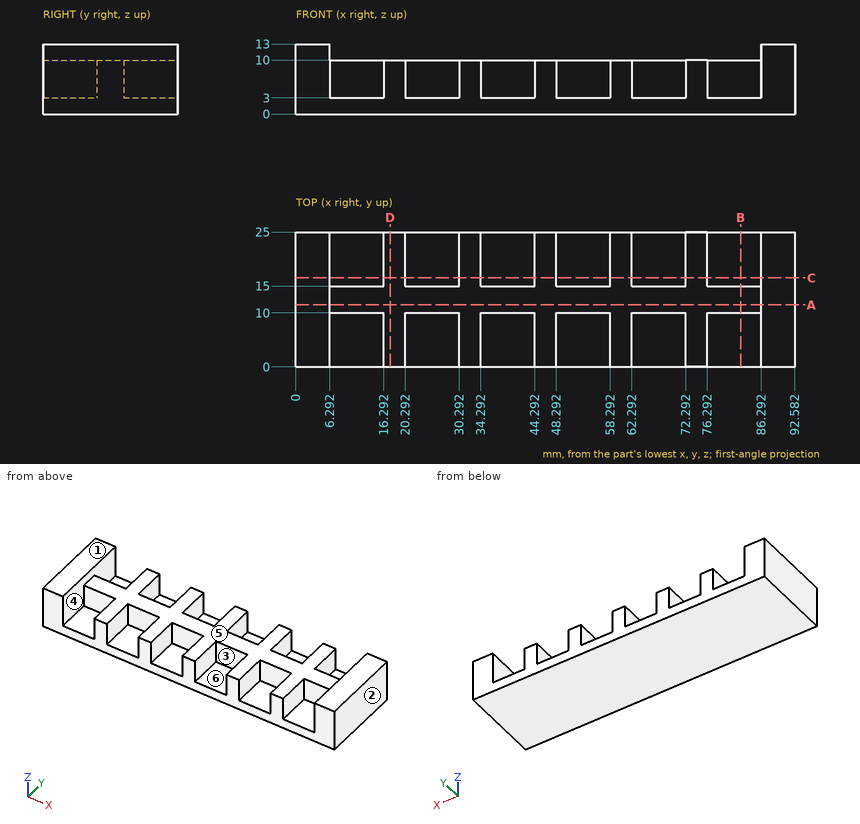
Part print with two shaded views. Sizes in mm from the minimum x, y, z corner. A direction names the side the tool comes from. Coordinates: 2 decimals unless noted, no trailing zeros. Order: outer loops, then holes, each group sorted by start corner. A loop starts at its lowest first (then second) coordinate and runs counter-clockwise, first axis right, second up.
(1) Saw through at D-D, the plane x = 17.5. Write the cut outline in (y, z).
Solution:
outline: (0, 0) - (25, 0) - (25, 10) - (0, 10) - close
(2) Saw through at C-C, the plane y = 16.5. Write the cut outline in (x, z).
Solution:
outline: (0, 0) - (92.58, 0) - (92.58, 13) - (86.29, 13) - (86.29, 3) - (76.29, 3) - (76.29, 10) - (72.29, 10) - (72.29, 3) - (62.29, 3) - (62.29, 10) - (58.29, 10) - (58.29, 3) - (48.29, 3) - (48.29, 10) - (44.29, 10) - (44.29, 3) - (34.29, 3) - (34.29, 10) - (30.29, 10) - (30.29, 3) - (20.29, 3) - (20.29, 10) - (16.29, 10) - (16.29, 3) - (6.29, 3) - (6.29, 13) - (0, 13) - close
(3) Pin check, flat tips, straight feed: pin 1 Ø8 at (x, y) = (11.5, 5.5) entering from +Z; pin 2 Ø5 at (x, z) = (55.5, 8) entering from +Y; pin 3 Ø8 at (x, y) = (79, 5) entering from +Z. Stop position of each tip, or through.
Solution:
pin 1: stops at z = 3
pin 2: stops at y = 15
pin 3: stops at z = 10
(4) Which spindle directions (+Z, -Z, +X, -X, +Y, -Y) get a long thin tool onto all of the face, cutting with end or side? Do the marked faces 4, 5 and 6. Say none if no direction does.
Solution:
face 4: +Z
face 5: +Z, +Y, -Y
face 6: +Z, -Y
(5) Saw through at A-A, the plane y = 11.5. Write the cut outline in (x, z).
Solution:
outline: (0, 0) - (92.58, 0) - (92.58, 13) - (86.29, 13) - (86.29, 10) - (6.29, 10) - (6.29, 13) - (0, 13) - close
(6) Mould opens along X. For the marked faces 1, 2 and 3 say: released by +X, released by -X, zero draft, split by the parting line, or undercut.
Solution:
face 1: zero draft
face 2: released by +X
face 3: undercut
(7) Drill centre lines: L1, parallel to X at y = 4, z = 10.5; L2, parallel to Z at x = 8, y = 19; L3, parallel to Y at x = 80, z = 7.75. Where is each one in solid material? Low to high.
Solution:
L1: x = 0 to 6.29, 86.29 to 92.58
L2: z = 0 to 3
L3: y = 10 to 15
(8) Saw through at B-B, the plane x = 82.5. Write the cut outline in (y, z), and give its area (3 significant figures).
Solution:
outline: (0, 0) - (25, 0) - (25, 3) - (15, 3) - (15, 10) - (10, 10) - (10, 3) - (0, 3) - close
area: 110 mm2
